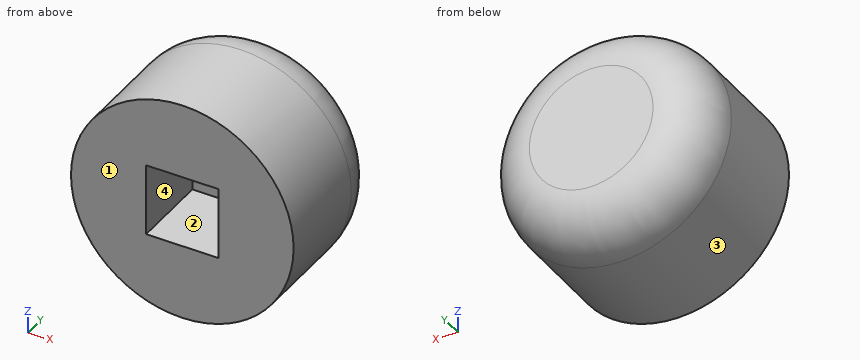
```python
from build123d import *

# Parameters (mm, degrees)
SKETCH_1_R          = 11.25
EXTRUDE_1_DEPTH     = 15
FILLET_1_R          = 5
SKETCH_2_W          = 7.3
SKETCH_2_H          = 7.3
CUT_EXTRUDE_1_DEPTH = 8


with BuildPart() as part:
    # 草图1 → 凸台-拉伸1 (new body)
    with BuildSketch(Plane(origin=(0, 0, 0), x_dir=(1, 0, 0), z_dir=(0, 1, 0))):
        with Locations(Location((0, 0, 0), (0, 0, 270))):
            Circle(SKETCH_1_R)
    extrude(amount=EXTRUDE_1_DEPTH)

    # 圆角1
    fillet_1_edges = [part.edges().sort_by_distance(p)[0] for p in [
        (0, 15, -11.25),
    ]]
    fillet(fillet_1_edges, radius=FILLET_1_R)

    # 草图2 → 切除-拉伸1 (cut)
    with BuildSketch(Plane.XZ):
        Rectangle(SKETCH_2_W, SKETCH_2_H)
    extrude(amount=-CUT_EXTRUDE_1_DEPTH, mode=Mode.SUBTRACT)


solid = part.part
```
Could you check a few things on this model? Use its own coordinates, in mm. Face numbers are marked on the shaded views. Round coordinates to 2 decimals unless told otherwise and drop trailing zeros. Write each loop counter-clockwise with the first axis right and the second up, starting at its lowest first coordinate (ties: lowest second). Pieces come first, ordered by that corner, then holes. Notation, with made-up numbers: M -7.5,55.25 L 38.5,55.25 A26 cw 38.5,69.25 Z; hole C -1.75,47 d3. An arc over 180 degrees is marked long. Write each question's results on one line, items separated by ' | '. Start each with the question number.
1. Imagine slicing it at D-D on y = 8.5. List the corners of the cut face in (x, z) for me, and give its area (3 significant figures).
2. Imagine slicing it at B-B on z = 0. List the corners of the cut face in (x, y) for me, and give its area (3 significant figures).
3. I need wall thicknesses on L1, parallel to Y at x = -2.25, z = 2; L2, parallel to Z at x = -2.5, y = 3.5; L3, parallel to Z at x = 1, y = 5.5. Which ranges of each line are inside material? Lowest first, please. Write a range as from..to.
4. Thinking about a two-plate mould opening in Z: for the marked faces 1, 2, 3 and 4, which applies, +Z half, -Z half, draft (parallel to the pull), parting line (faces both ways), or undercut?
5. Imagine slicing it at C-C on x = 0. List the corners of the cut face in (y, z) for me, and give its area (3 significant figures).
6. I'm going to push flat-ended pins straight in: pin 1 Ø6 at (y, z) = (11, 7.5) entering from +X; pin 2 Ø2 at (x, z) = (-7, 7.5) entering from +Y. Where does each tip first touch, or does it pass through?
7. Imagine slicing it at A-A on y = 6. List the corners of the cut face in (x, z) for me.
Result sheet:
1) outline: C 0,0 d22.5 | area: 398 mm^2
2) outline: M -11.25,0 L -3.65,0 L -3.65,8 L 3.65,8 L 3.65,0 L 11.25,0 L 11.25,10 A5 ccw 6.25,15 L -6.25,15 A5 ccw -11.25,10 Z | area: 268 mm^2
3) L1: y = 8..15 | L2: z = -10.97..-3.65, 3.65..10.97 | L3: z = -11.21..-3.65, 3.65..11.21
4) face 1: draft | face 2: undercut | face 3: parting line | face 4: undercut
5) outline: M 0,-11.25 L 10,-11.25 A5 ccw 15,-6.25 L 15,6.25 A5 ccw 10,11.25 L 0,11.25 L 0,3.65 L 8,3.65 L 8,-3.65 L 0,-3.65 Z | area: 268 mm^2
6) pin 1: stops at x = 10.27 | pin 2: stops at y = 13.99
7) outline: C 0,0 d22.5; hole M -3.65,-3.65 L 3.65,-3.65 L 3.65,3.65 L -3.65,3.65 Z
